For this review, take the finished solid that the model builds, in its own axes (mm). A direction names the side the tool comes from. Round coordinates to 2 decimals unless told otherwise and drop trailing zeros. Order: outer loops, then holes, each group sorted by start corner. A loop starts at its lowest first (then second) coordinate and runs counter-clockwise, first axis right, second up.
```python
from build123d import *

# Parameters (mm, degrees)
F1_DEPTH       = 30
F2_R           = 5
F4_START       = -28
F4_DEPTH       = 28.001
F6_D           = 5
F6_CBORE_D     = 9
F6_CBORE_DEPTH = 1.5
F7_D           = 12
F7_DEPTH       = 52.001


with BuildPart() as f1:
    # F0 (on Top) → F1 (new body)
    with BuildSketch(Plane.XY):
        with BuildLine():
            ThreePointArc((7, 24), (0, -25), (-7, 24))
            Line((-7, 24), (-14.4222051019, 24))
            ThreePointArc((-14.4222051019, 24), (0, -28), (14.4222051019, 24))
            Line((14.4222051019, 24), (7, 24))
        make_face()
        Polygon((-14.4222051019, 24), (-7, 24), (7, 24), (14.4222051019, 24), (28, 24), (28, 28), (-28, 28), (-28, 24), align=None)
    extrude(amount=F1_DEPTH)

    # F2
    f2_edges = [f1.edges().sort_by_distance(p)[0] for p in [
        (-14.422205, 24, 15),
        (14.422205, 24, 15),
    ]]
    fillet(f2_edges, radius=F2_R)

    # F3 (on face) → F4 (cut)
    with BuildSketch(Plane(origin=(0, 28, 0), x_dir=(-1, 0, 0), z_dir=(0, 1, 0)).offset(F4_START)):
        Polygon((28, 30), (16, 30), (-28, 0), (-16, 0), align=None)
    extrude(amount=-F4_DEPTH, mode=Mode.SUBTRACT)

    # F6 (through all)
    with Locations(Plane.XZ.offset(-24)):
        with Locations((0, 15)):
            CounterBoreHole(F6_D / 2, F6_CBORE_D / 2, F6_CBORE_DEPTH)

    # F7 (through all, one way)
    with BuildSketch(Plane(origin=(0, 24, 0), x_dir=(1, 0, 0), z_dir=(0, 1, 0))):
        with Locations((0, -15)):
            Circle(F7_D / 2)
    extrude(amount=-F7_DEPTH, mode=Mode.SUBTRACT)


solid = f1.part
```
Q1. Clearance check with flat-ended pins moving along their axes: pin 1 (1 mm diameter, centred on y = 0.5, z = 24.5, fed in from +X); pin 2 (7 mm diameter, centred on x = -3, z = 15.5, fed in from -Y); pin 3 (1 mm diameter, centred on x = 26, z = 0.5, fed in from -Y). State where each tip first meets the part, or that it passes through.
Q2. Wall thickness on line 1 (X direction, y = 0, z = 7); line 2 (Y direction, x = 0, z = 8.5); line 3 (Y direction, x = 23, z = 11): over which ranges is each line inside the solid? List them lowest first.
Q3. Take a section at B-B, the plane y = 21.5. State the section outline as (x, z) points, plus the area to 3 significant figures.
Q4. Tool access review of faces 4 (the face through (0.54, 26.77, 12.56)), 5 (the face through (-20.21, -15.64, 24.69)), 6 (the face through (-24.82, -2.98, 11.46)), 7 (the face through (26, 0, 1)), 8 (the face through (9.128, -24.509, 4.685)): name each direction out of +Z, -Z, +X, -X, +Y, -Y from which nothing blocks a thin tool from reaching the whole face with its end or side.
Q5. Take a section at D-D, the plane z = 3. State the section outline as (x, y) points.
Q6. Take a section at A-A, the plane x = 0. State the section outline as (y, z) points.
Q7. Mouldability with a two-part tool opening along Z and no side actions: class faces 1 (the face through (2.419, 24.74, 18.794)), 2 (the face through (2, 25, 30)), 3 (the face through (-26, 0, 29)) as +Z half, -Z half, draft (parallel to the pull), parting line (faces both ways), or undercut.
Q8. Take a section at C-C, the plane x = -19. State the section outline as (y, z) points, plus the area to 3 significant figures.
Working result:
1. pin 1: stops at x = 28
1. pin 2: stops at y = -27.4
1. pin 3: stops at y = 0
2. line 1: x = -28 to -25, 25 to 28
2. line 2: y = -28 to -25, 24 to 28
2. line 3: y = -15.97 to -9.8, 9.8 to 15.97, 22.02 to 28
3. outline: (-22.65, 0) - (-12.76, 0) - (-12.76, 30) - (-22.65, 30) - close; (12.76, 0) - (22.65, 0) - (22.65, 30) - (12.76, 30) - close
3. area: 594 mm2
4. face 4: +Y, -Y
4. face 5: -Y
4. face 6: +Z, -Z
4. face 7: -Z, -Y
4. face 8: +X, -Y
5. outline: (-28, 24) - (-26.98, 24) arc R5 cw to (-22.89, 16.12) arc R28 ccw to (11.6, -25.48) - (11.6, -22.15) arc R25 cw (long way) to (-7, 24) - (7, 24) arc R25 cw to (23.6, -8.25) - (23.6, -15.07) arc R28 ccw to (22.89, 16.12) arc R5 cw to (26.98, 24) - (28, 24) - (28, 28) - (-28, 28) - close
6. outline: (-28, 0) - (-25, 0) - (-25, 9) - (-28, 9) - close; (-28, 21) - (-25, 21) - (-25, 30) - (-28, 30) - close; (24, 0) - (28, 0) - (28, 12.5) - (25.5, 12.5) - (25.5, 10.5) - (24, 10.5) - close; (24, 19.5) - (25.5, 19.5) - (25.5, 17.5) - (28, 17.5) - (28, 30) - (24, 30) - close
7. face 1: undercut
7. face 2: +Z half
7. face 3: draft
8. outline: (-20.57, 0) - (-16.25, 0) - (-16.25, 23.86) - (-20.57, 23.86) - close; (16.25, 0) - (28, 0) - (28, 30) - (16.25, 30) - close
8. area: 456 mm2
